```python
from build123d import *

# Parameters (mm, degrees)
SKIZZE1_W                            = 60
SKIZZE1_H                            = 80
SKIZZE1_R                            = 1.65
SKIZZE1_R_2                          = 6.25
AUFSATZ_LINEAR_AUSTRAGEN1_DEPTH      = 5
VERRUNDUNG1_SIZE                     = 15
VERRUNDUNG1_SIZE_2                   = 20
AUFSATZ_LINEAR_AUSTRAGEN2_DEPTH      = 11
AUFSATZ_LINEAR_AUSTRAGEN2_DEPTH_BACK = 16
SKIZZE2_W                            = 60
SKIZZE2_H                            = 12.5
SCHNITT_LINEAR_AUSTRAGEN1_DEPTH      = 13
SCHNITT_LINEAR_AUSTRAGEN2_DEPTH      = 0.5
SCHNITT_LINEAR_AUSTRAGEN2_DEPTH_BACK = 13
SKIZZE4_W                            = 10.5
SKIZZE4_H                            = 10.5


with BuildPart() as part:
    # Skizze1 → Aufsatz-Linear austragen1 (new body)
    with BuildSketch(Plane.XY):
        Rectangle(SKIZZE1_W, SKIZZE1_H)
        with Locations((-5, 35)):
            Circle(SKIZZE1_R, mode=Mode.SUBTRACT)
        with Locations((5, 35)):
            Circle(SKIZZE1_R, mode=Mode.SUBTRACT)
        with Locations((-18.488104712, 12.772291363)):
            Circle(SKIZZE1_R_2, mode=Mode.SUBTRACT)
        with Locations((18.488104712, 12.772291363)):
            Circle(SKIZZE1_R_2, mode=Mode.SUBTRACT)
    extrude(amount=AUFSATZ_LINEAR_AUSTRAGEN1_DEPTH)

    # Verrundung1
    # a fillet whose section is not a circle: 20, 15 mm, written as the material it takes off along each edge
    with BuildSketch(Plane(origin=(30, 40, -50), x_dir=(0, -1, 0), z_dir=(0, 0, 1))) as verrundung1_piece_1:
        with BuildLine():
            Bezier((VERRUNDUNG1_SIZE, 0), (0, 0), (0, -VERRUNDUNG1_SIZE_2), weights=[1, 1, 1])
            Line((0, -VERRUNDUNG1_SIZE_2), (0, 0))
            Line((0, 0), (VERRUNDUNG1_SIZE, 0))
        make_face()
    extrude(amount=105, mode=Mode.SUBTRACT)
    with BuildSketch(Plane(origin=(-30, 40, -50), x_dir=(1, 0, 0), z_dir=(0, 0, 1))) as verrundung1_piece_2:
        with BuildLine():
            Bezier((VERRUNDUNG1_SIZE_2, 0), (0, 0), (0, -VERRUNDUNG1_SIZE), weights=[1, 1, 1])
            Line((0, -VERRUNDUNG1_SIZE), (0, 0))
            Line((0, 0), (VERRUNDUNG1_SIZE_2, 0))
        make_face()
    extrude(amount=105, mode=Mode.SUBTRACT)

    # Skizze2 → Aufsatz-Linear austragen2 (add, two sides: drawn at the far end of the back side and taken through both)
    with BuildSketch(Plane.XY.offset(5).offset(-AUFSATZ_LINEAR_AUSTRAGEN2_DEPTH_BACK)):
        with Locations((0, -33.75)):
            Rectangle(SKIZZE2_W, SKIZZE2_H)
    extrude(amount=AUFSATZ_LINEAR_AUSTRAGEN2_DEPTH + AUFSATZ_LINEAR_AUSTRAGEN2_DEPTH_BACK)

    # Skizze3 → Schnitt-Linear austragen1 (cut)
    with BuildSketch(Plane.XZ.offset(40)):
        with BuildLine():
            Line((2.8, 4.05), (2.8, 0.95))
            Line((2.8, 0.95), (3.687478813, 0.95))
            ThreePointArc((3.687478813, 0.95), (3.921091382, 1.709403786), (4, 2.5))
            ThreePointArc((4, 2.5), (3.921091382, 3.290596214), (3.687478813, 4.05))
            Line((3.687478813, 4.05), (2.8, 4.05))
        make_face()
        with BuildLine():
            Line((3.687478813, 0.95), (2.8, 0.95))
            Line((2.8, 0.95), (2.8, 4.05))
            Line((2.8, 4.05), (3.687478813, 4.05))
            ThreePointArc((3.687478813, 4.05), (-4, 2.5), (3.687478813, 0.95))
        make_face()
        with BuildLine():
            ThreePointArc((4, 2.5), (3.921091382, 1.709403786), (3.687478813, 0.95))
            Line((3.687478813, 0.95), (5.2, 0.95))
            Line((5.2, 0.95), (5.2, 4.05))
            Line((5.2, 4.05), (3.687478813, 4.05))
            ThreePointArc((3.687478813, 4.05), (3.921091382, 3.290596214), (4, 2.5))
        make_face()
    extrude(amount=-SCHNITT_LINEAR_AUSTRAGEN1_DEPTH, mode=Mode.SUBTRACT)

    # Skizze4 → Schnitt-Linear austragen2 (cut, two sides: drawn at the far end of the back side and taken through both)
    with BuildSketch(Plane.XZ.offset(27).offset(-SCHNITT_LINEAR_AUSTRAGEN2_DEPTH_BACK)):
        with Locations((0, 2.5)):
            Rectangle(SKIZZE4_W, SKIZZE4_H)
    extrude(amount=SCHNITT_LINEAR_AUSTRAGEN2_DEPTH + SCHNITT_LINEAR_AUSTRAGEN2_DEPTH_BACK, mode=Mode.SUBTRACT)


solid = part.part
```
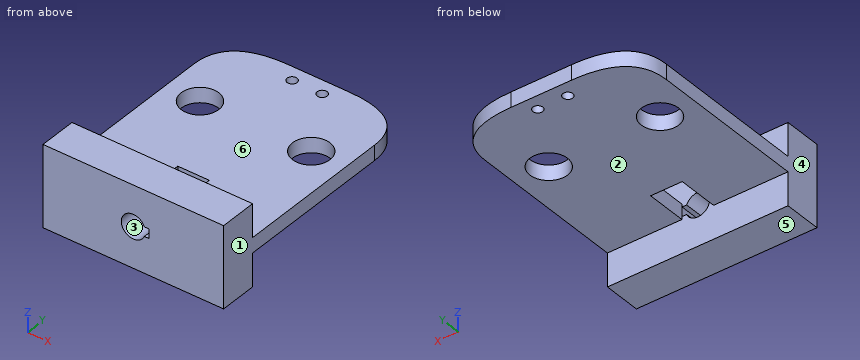
Input: part model. Units: mm. Frame: model coordinates. Face numbers are marked on the shaded views. A direction names the side the tool comes from. Give positions to 0.01 mm unless a question says otherwise; leave off trailing zeros. Order: outer loops, then holes, each group sorted by start corner. A loop starts at its lowest first (then second) coordinate and runs counter-clockwise, first axis right, second up. Notation, with made-up numbers: (17, 28) - (60, 28) arc R8 cw to (60, 34) - close; hole circle Ø5 at (-39.75, -34.5). An arc over 180 degrees is marked (long way). Put each result on its own line as item: value.
Item 1: Ray query, L1, parallel to Z at x = 4.5, y = -35; L2, parallel to Z at x = 0, y = -30; L3, parallel to Y at x = 25.5, z = 11. Return the intervals inside material, ascending. Write a range as from..to.
Found:
L1: z = -11..0.95, 4.05..16
L2: z = -11..-1.5, 6.5..16
L3: y = -40..-27.5
Item 2: Section query C-C, the plane z = 11.25. Return loops of the section in (x, y), then the cut area to 3 significant figures.
Found:
outline: (-30, -40) - (30, -40) - (30, -27.5) - (-30, -27.5) - close
area: 750 mm^2
Item 3: Access query for the marked faces 5 and 6. Directions: +Z, -Z, +X, -X, +Y, -Y. A direction counts if a zero-diameter tool reaches every point of the face in a straight line with its end or side. Return the directions, or none.
Found:
face 5: -Z, +X, -X, +Y, -Y
face 6: +Z, +X, -X, +Y
Item 4: Draft query along X for the marked faces 1, 2, 3 and 4. Return one class per face: +X half, -X half, draft (parallel to the pull), parting line (faces both ways), or undercut.
Found:
face 1: +X half
face 2: draft
face 3: undercut
face 4: -X half
Item 5: Section query B-B, the plane y = -29. Return loops of the section in (x, z), then the cut area to 3 significant figures.
Found:
outline: (-30, -11) - (30, -11) - (30, 16) - (-30, 16) - close; hole (3.69, 0.95) - (5.2, 0.95) - (5.2, 4.05) - (3.69, 4.05) arc R4 ccw (long way) to start
area: 1,570 mm^2
Item 6: Section query D-D, the plane y = 3. Return loops of the section in (x, z).
Found:
outline: (-30, 0) - (30, 0) - (30, 5) - (-30, 5) - close
Item 7: Contact query for flat-ended pins moving along their axis: pin 1 (2 mm diameter, centred on x = 23.5, y = 26.5, fed in from -Z); pin 2 (5.5 mm diameter, centred on x = -0.5, z = 2.5, fed in from -Y); pin 3 (14.5 mm diameter, centred on x = 18.49, y = 12.77, fed in from +Z). Output: stop coordinate, or through.
Found:
pin 1: stops at z = 0
pin 2: stops at y = -14
pin 3: stops at z = 5
Item 8: Section query A-A, the plane x = 0. Return loops of the section in (y, z), then the cut area to 4 significant figures.
Found:
outline: (-40, -11) - (-27.5, -11) - (-27.5, -1.5) - (-40, -1.5) - close; (-40, 6.5) - (-27.5, 6.5) - (-27.5, 16) - (-40, 16) - close; (-14, 0) - (40, 0) - (40, 5) - (-14, 5) - close
area: 507.5 mm^2
